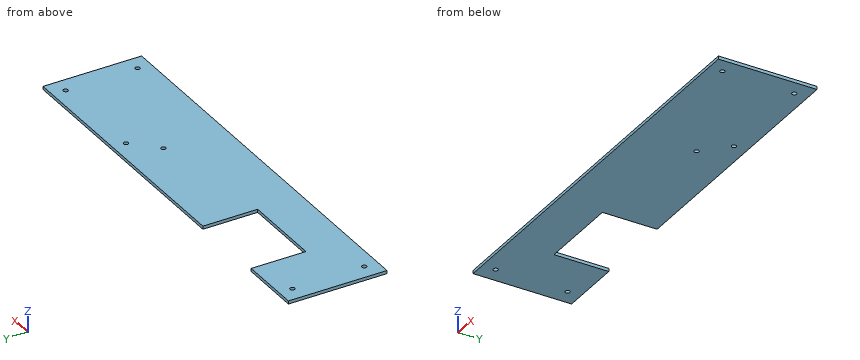
```python
from build123d import *

# Parameters (mm, degrees)
ESQUISSE1_W      = 264
ESQUISSE1_H      = 63
ESQUISSE1_R      = 1.5
EXTRUSION1_DEPTH = 2
ESQUISSE2_R      = 1.5
EXTRUSION2_DEPTH = 10
ESQUISSE3_W      = 52
ESQUISSE3_H      = 35
EXTRUSION3_DEPTH = 10


with BuildPart() as part:
    # Esquisse1 → Extrusion1 (new body)
    with BuildSketch(Plane.XY):
        with Locations((86.261300687, 18.408191489)):
            Rectangle(ESQUISSE1_W, ESQUISSE1_H)
        with Locations((-35.738699313, 41.408191489)):
            Circle(ESQUISSE1_R, mode=Mode.SUBTRACT)
        with Locations((-35.738699313, -4.591808511)):
            Circle(ESQUISSE1_R, mode=Mode.SUBTRACT)
        with Locations((208.261300687, 41.408191489)):
            Circle(ESQUISSE1_R, mode=Mode.SUBTRACT)
        with Locations((208.261300687, -4.591808511)):
            Circle(ESQUISSE1_R, mode=Mode.SUBTRACT)
    extrude(amount=EXTRUSION1_DEPTH)

    # Esquisse2 → Extrusion2 (cut)
    with BuildSketch(Plane.XY.offset(2)):
        with Locations((143.261300687, 41.408191489)):
            Circle(ESQUISSE2_R)
        with Locations((128.261300687, 26.408191489)):
            Circle(ESQUISSE2_R)
    extrude(amount=-EXTRUSION2_DEPTH, mode=Mode.SUBTRACT)

    # Esquisse3 → Extrusion3 (cut)
    with BuildSketch(Plane.XY.offset(2)):
        with Locations((20.261300687, 32.408191489)):
            Rectangle(ESQUISSE3_W, ESQUISSE3_H)
    extrude(amount=-EXTRUSION3_DEPTH, mode=Mode.SUBTRACT)


solid = part.part
```
Part model, mm, in its own coordinate system. Give positions to 0.01 mm unless a question says otherwise; leave off trailing zeros. Write each loop counter-clockwise with the first axis right and the second up, starting at its lowest first coordinate (ties: lowest second). Pieces come first, ordered by that corner, then holes. Notation, with made-up numbers: (-29.75, 38.5) -> (-22.75, 38.5) arc R21 ccw to (-22.75, 69.5) -> close; hole circle Ø10 at (14.5, -33.5). An arc over 180 degrees is marked (long way). Put each result on its own line as item: value. Start each with the question number.
Item 1: Wall check: L1, parallel to X at y = 18.5, z = 1.1; L2, parallel to X at y = -5, z = 0.7; L3, parallel to X at y = -5.5, z = 0.55. Give the ranges that are in metal, low to high. Write a range as [from, to].
Item 2: Pin check, flat tip, straight feed: pin 1 Ø1 at (x, z) = (15, 0.5) entering from +Y. Stop position of the tip, or through.
Item 3: Cut at B-B (x = 7.5). List the corners of the cut face in (y, z).
Item 4: Cut at A-A (z = 0.9). List the corners of the cut face in (x, y), then the cut area to 3 significant figures.
Answer list:
1. L1: x = [-45.74, -5.74], [46.26, 218.26]
1. L2: x = [-45.74, -37.18], [-34.3, 206.82], [209.7, 218.26]
1. L3: x = [-45.74, -36.93], [-34.54, 207.07], [209.46, 218.26]
2. pin 1: stops at y = 14.91
3. outline: (-13.09, 0) -> (14.91, 0) -> (14.91, 2) -> (-13.09, 2) -> close
4. outline: (-45.74, -13.09) -> (218.26, -13.09) -> (218.26, 49.91) -> (46.26, 49.91) -> (46.26, 14.91) -> (-5.74, 14.91) -> (-5.74, 49.91) -> (-45.74, 49.91) -> close; hole circle Ø3 at (-35.74, -4.59); hole circle Ø3 at (-35.74, 41.41); hole circle Ø3 at (128.26, 26.41); hole circle Ø3 at (143.26, 41.41); hole circle Ø3 at (208.26, -4.59); hole circle Ø3 at (208.26, 41.41)
4. area: 14,800 mm2
